```python
from build123d import *

# Parameters (mm, degrees)
CROQUIS2_R              = 16
SALIENTE_EXTRUIR1_DEPTH = 6
CROQUIS3_R              = 2.7
SALIENTE_EXTRUIR2_DEPTH = 50
CROQUIS4_R              = 2.7
CROQUIS4_R_2            = 2
CORTAR_EXTRUIR1_DEPTH   = 5


with BuildPart() as part:
    # Croquis2 → Saliente-Extruir1 (new body)
    with BuildSketch(Plane.XY):
        Circle(CROQUIS2_R)
        with BuildLine():
            Line((1.25, 12.165063509), (1.25, 11.25))
            Line((1.25, 11.25), (2.165063509, 11.25))
            ThreePointArc((2.165063509, 11.25), (2.414814566, 10.647047613), (2.5, 10))
            ThreePointArc((2.5, 10), (2.414814566, 9.352952387), (2.165063509, 8.75))
            Line((2.165063509, 8.75), (1.25, 8.75))
            Line((1.25, 8.75), (1.25, 7.834936491))
            ThreePointArc((1.25, 7.834936491), (0.647047613, 7.585185434), (0, 7.5))
            ThreePointArc((0, 7.5), (-0.647047613, 7.585185434), (-1.25, 7.834936491))
            Line((-1.25, 7.834936491), (-1.25, 8.75))
            Line((-1.25, 8.75), (-2.165063509, 8.75))
            ThreePointArc((-2.165063509, 8.75), (-2.414814566, 9.352952387), (-2.5, 10))
            ThreePointArc((-2.5, 10), (-2.414814566, 10.647047613), (-2.165063509, 11.25))
            Line((-2.165063509, 11.25), (-1.25, 11.25))
            Line((-1.25, 11.25), (-1.25, 12.165063509))
            ThreePointArc((-1.25, 12.165063509), (-0.647047613, 12.414814566), (0, 12.5))
            ThreePointArc((0, 12.5), (0.647047613, 12.414814566), (1.25, 12.165063509))
        make_face(mode=Mode.SUBTRACT)
        with BuildLine():
            Line((12.165063509, -1.25), (11.25, -1.25))
            Line((11.25, -1.25), (11.25, -2.165063509))
            ThreePointArc((11.25, -2.165063509), (10.647047613, -2.414814566), (10, -2.5))
            ThreePointArc((10, -2.5), (9.352952387, -2.414814566), (8.75, -2.165063509))
            Line((8.75, -2.165063509), (8.75, -1.25))
            Line((8.75, -1.25), (7.834936491, -1.25))
            ThreePointArc((7.834936491, -1.25), (7.585185434, -0.647047613), (7.5, 0))
            ThreePointArc((7.5, 0), (7.585185434, 0.647047613), (7.834936491, 1.25))
            Line((7.834936491, 1.25), (8.75, 1.25))
            Line((8.75, 1.25), (8.75, 2.165063509))
            ThreePointArc((8.75, 2.165063509), (9.352952387, 2.414814566), (10, 2.5))
            ThreePointArc((10, 2.5), (10.647047613, 2.414814566), (11.25, 2.165063509))
            Line((11.25, 2.165063509), (11.25, 1.25))
            Line((11.25, 1.25), (12.165063509, 1.25))
            ThreePointArc((12.165063509, 1.25), (12.414814566, 0.647047613), (12.5, 0))
            ThreePointArc((12.5, 0), (12.414814566, -0.647047613), (12.165063509, -1.25))
        make_face(mode=Mode.SUBTRACT)
        with BuildLine():
            Line((-1.25, -12.165063509), (-1.25, -11.25))
            Line((-1.25, -11.25), (-2.165063509, -11.25))
            ThreePointArc((-2.165063509, -11.25), (-2.414814566, -10.647047613), (-2.5, -10))
            ThreePointArc((-2.5, -10), (-2.414814566, -9.352952387), (-2.165063509, -8.75))
            Line((-2.165063509, -8.75), (-1.25, -8.75))
            Line((-1.25, -8.75), (-1.25, -7.834936491))
            ThreePointArc((-1.25, -7.834936491), (-0.647047613, -7.585185434), (0, -7.5))
            ThreePointArc((0, -7.5), (0.647047613, -7.585185434), (1.25, -7.834936491))
            Line((1.25, -7.834936491), (1.25, -8.75))
            Line((1.25, -8.75), (2.165063509, -8.75))
            ThreePointArc((2.165063509, -8.75), (2.414814566, -9.352952387), (2.5, -10))
            ThreePointArc((2.5, -10), (2.414814566, -10.647047613), (2.165063509, -11.25))
            Line((2.165063509, -11.25), (1.25, -11.25))
            Line((1.25, -11.25), (1.25, -12.165063509))
            ThreePointArc((1.25, -12.165063509), (0.647047613, -12.414814566), (0, -12.5))
            ThreePointArc((0, -12.5), (-0.647047613, -12.414814566), (-1.25, -12.165063509))
        make_face(mode=Mode.SUBTRACT)
        with BuildLine():
            Line((-12.165063509, 1.25), (-11.25, 1.25))
            Line((-11.25, 1.25), (-11.25, 2.165063509))
            ThreePointArc((-11.25, 2.165063509), (-10.647047613, 2.414814566), (-10, 2.5))
            ThreePointArc((-10, 2.5), (-9.352952387, 2.414814566), (-8.75, 2.165063509))
            Line((-8.75, 2.165063509), (-8.75, 1.25))
            Line((-8.75, 1.25), (-7.834936491, 1.25))
            ThreePointArc((-7.834936491, 1.25), (-7.585185434, 0.647047613), (-7.5, 0))
            ThreePointArc((-7.5, 0), (-7.585185434, -0.647047613), (-7.834936491, -1.25))
            Line((-7.834936491, -1.25), (-8.75, -1.25))
            Line((-8.75, -1.25), (-8.75, -2.165063509))
            ThreePointArc((-8.75, -2.165063509), (-9.352952387, -2.414814566), (-10, -2.5))
            ThreePointArc((-10, -2.5), (-10.647047613, -2.414814566), (-11.25, -2.165063509))
            Line((-11.25, -2.165063509), (-11.25, -1.25))
            Line((-11.25, -1.25), (-12.165063509, -1.25))
            ThreePointArc((-12.165063509, -1.25), (-12.414814566, -0.647047613), (-12.5, 0))
            ThreePointArc((-12.5, 0), (-12.414814566, 0.647047613), (-12.165063509, 1.25))
        make_face(mode=Mode.SUBTRACT)
    extrude(amount=SALIENTE_EXTRUIR1_DEPTH)

    # Croquis3 → Saliente-Extruir2 (add)
    with BuildSketch(Plane(origin=(0, 0, 0), x_dir=(-1, 0, 0), z_dir=(0, 0, -1))):
        Circle(CROQUIS3_R)
    extrude(amount=SALIENTE_EXTRUIR2_DEPTH)

    # Croquis4 → Cortar-Extruir1 (cut)
    with BuildSketch(Plane(origin=(0, 0, -50), x_dir=(-1, 0, 0), z_dir=(0, 0, -1))):
        Circle(CROQUIS4_R)
        Circle(CROQUIS4_R_2, mode=Mode.SUBTRACT)
    extrude(amount=-CORTAR_EXTRUIR1_DEPTH, mode=Mode.SUBTRACT)


solid = part.part
```
The listing builds one solid part. Answer for the finished solid, in the listing's coordinates (mm). A direction names the side the tool comes from. Round coordinates to 2 decimals unless told otherwise and drop trailing zeros. Loops run counter-clockwise (first coordinate to the right, second up) from the corner with the lowest first, then second, coordinate; pieces in that order, holes last. Notation, with made-up numbers: (14, 48.25) - (32, 48.25) arc R21 ccw to (32, 64.25) - close; hole circle Ø4 at (54, 59.5). An arc over 180 degrees is marked (long way). Return JSON: item names as keys, results as strings. Group by question number.
1. Each of these flat-tipped pins is pushed along its axis until it touches: P1, Ø1, axis at y = 2, z = 2, coming from the +X side; P2, Ø1.5, axis at x = -2.5, y = -11.5, coming from the -Z side; P3, Ø0.5, axis at y = -8.5, z = 3.5, coming from the +X side. Where does it stop, or does it pass through?
2. The part is cut by section A-A on z = -42. Determine the outline of the cut face in (x, y).
3. Which of the six approach directions +Z, -Z, +X, -X, +Y, -Y give full straight-line access (tool end or side, diameter ignored) to faces 1 (the cylindrical face through (0, -2, -48)), 2 (the flat face through (0, 0, 6))?
4. The part is cut by section B-B on x = -6. Determine the outline of the cut face in (y, z), then the cut area to 3 significant figures.
5. Consider probe 1 along Z at (x, y) = (6, -5); probe 2 along X at (y, z) = (-1, -24.5); probe 3 along X at (y, z) = (8.5, 2). Determine where each line is inside the solid, lowest interval first.
Resolved:
{
 "1": {"P1": "stops at x = 15.93", "P2": "stops at z = 0", "P3": "stops at x = 13.71"},
 "2": {"outline": "circle Ø5.4 at (0, 0)"},
 "3": {"face 1": "-Z", "face 2": "+Z, +X, -X, +Y, -Y"},
 "4": {"outline": "(-14.83, 0) - (14.83, 0) - (14.83, 6) - (-14.83, 6) - close", "area": "178 mm²"},
 "5": {"probe 1": "z = 0 to 6", "probe 2": "x = -2.51 to 2.51", "probe 3": "x = -13.56 to -1.25, 1.25 to 13.56"}
}
